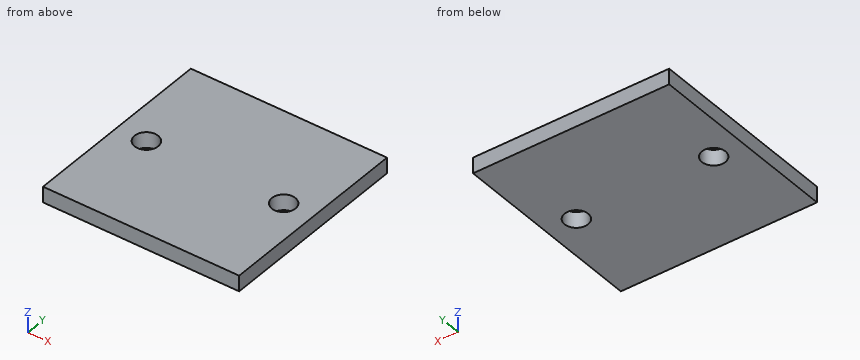
from build123d import *

# Parameters (mm, degrees)
F0_W     = 25
F0_H     = 25
F1_DEPTH = 2
F2_D     = 3


with BuildPart() as f1:
    # F0 (on Top) → F1 (new body)
    with BuildSketch(Plane.XY):
        Rectangle(F0_W, F0_H)
    extrude(amount=-F1_DEPTH)

    # F2 (through all)
    with Locations(Plane.XY):
        with Locations((-8.75, 0), (8.75, 0)):
            Hole(F2_D / 2)


solid = f1.part
CAD build for the part. Positions are in the model's coordinates, mm. Coordinates: 2 decimals unless noted, no trailing zeros. Write each loop counter-clockwise with the first axis right and the second up, starting at its lowest first coordinate (ties: lowest second). Pieces come first, ordered by that corner, then holes. Notation, with made-up numbers: (64, 81) - (87, 81) arc R30 ccw to (87, 117) - close; hole circle Ø9 at (-29.5, -39.75). An arc over 180 degrees is marked (long way). Use a Markdown table: item, result. Add a question column.
Item 1: Band-saw the part on C-C, the plane z = -0.5. Give the cut face in (x, y), and give its area (3 significant figures).
Item 2: Flat gauge pin, fed straight in: pin 1 (8 mm diameter, centred on x = -6, y = 9, fed in from +Z). Where does the tip first touch, or does it go through?
Item 3: Drill centre line: L1, parallel to Y at x = 8.75, z = -1.5. Where is it in solid material? Low to high. Write a range as from..to.
Item 4: Band-saw the part on B-B, the plane x = -8.75. Give the cut face in (y, z).
Item 5: Band-saw the part on A-A, the plane y = 0. Give the cut face in (x, z), and give its area (3 significant figures).
Numbers:
| question | item | result |
|---|---|---|
| 1 | outline | (-12.5, -12.5) - (12.5, -12.5) - (12.5, 12.5) - (-12.5, 12.5) - close; hole circle Ø3 at (-8.75, 0); hole circle Ø3 at (8.75, 0) |
| 1 | area | 611 mm2 |
| 2 | pin 1 | z = 0 |
| 3 | L1 | -12.5..-1.5, 1.5..12.5 |
| 4 | outline | (-12.5, -2) - (-1.5, -2) - (-1.5, 0) - (-12.5, 0) - close; (1.5, -2) - (12.5, -2) - (12.5, 0) - (1.5, 0) - close |
| 5 | outline | (-12.5, -2) - (-10.25, -2) - (-10.25, 0) - (-12.5, 0) - close; (-7.25, -2) - (7.25, -2) - (7.25, 0) - (-7.25, 0) - close; (10.25, -2) - (12.5, -2) - (12.5, 0) - (10.25, 0) - close |
| 5 | area | 38.0 mm2 |
